Read the model definition and answer for the solid it produces. Units are mm, in the model's axes. A direction names the side the tool comes from. Round coordinates to 2 decimals unless told otherwise and drop trailing zeros. Write each loop counter-clockwise with the first axis right and the second up, starting at its lowest first coordinate (ties: lowest second). Pieces come first, ordered by that corner, then holes. Notation, with made-up numbers: (-1, 44) -> (41, 44) arc R9 ccw to (41, 60) -> close; hole circle Ø5 at (48.25, 29.5). An arc over 180 degrees is marked (long way). Return JSON: item names as keys, results as strings. Group by question number.
(1) The mould has two halves that part along Z. Classify faces 3 (the cylindrical face through (4.032, -6.324, -11.888)), 4 (the flat face through (2, 5, -0.1)), 5 (the cylindrical face through (6.87, -2.16, -3.49)), 6 (the cylindrical face through (6.87, -2.16, -20.49)): released by +Z, released by -Z, zero draft, split by the parting line, or undercut.
(2) For faces 1 (the flat face through (-2, 5, -23.9)), 2 (the cylindrical face through (-0.867, 3.905, -12.168)), determine the directions among +Z, -Z, +X, -X, +Y, -Y from which every point of the face is accessible in a straight line to the end or side of a thin tool.
(3) Straight lines are drawn through the part: line 1 (Y direction, x = 0, z = -23.95); line 2 (Y direction, x = -0.25, z = -6.5); line 3 (Z direction, x = -3, y = -4.5). For each, find the intervals that lie inside material, in ascending order.
(4) A cutting plane is placed at A-A on z = -18.25. Give the vertices of the cut face in (x, y), then the cut area to 3 significant figures.
(5) Given pin 1 (1 mm diameter, centred on x = 3.5, y = 5, fed in from -Z); pin 2 (1.5 mm diameter, centred on x = -2, z = -9, fed in from +Y); pin 3 (3 mm diameter, centred on x = -3.5, z = -11, fed in from +Y); pin 4 (6 mm diameter, centred on y = -5, z = -21.5, fed in from +X), each flat-ended and moving along its own axis, determine where each tip first touches the part or whether it passes through.
```python
from build123d import *

# Parameters (mm, degrees)
FILLET1_R = 0.2


with BuildPart() as part:
    # Sketch1 → Revolve1 (revolve)
    with BuildSketch(Plane(origin=(0, 0, 0), x_dir=(0, 0, -1), z_dir=(1, 0, 0)), mode=Mode.PRIVATE) as revolve1_sk:
        Polygon((0, 7.5), (0, 6.5), (0.1, 6.5), (0.1, 5), (0, 5), (0, 4), (24, 4), (24, 5), (23.9, 5), (23.9, 6.5), (24, 6.5), (24, 7.5), (21, 7.5), (21, 7.2), (20, 7.2), (20, 7.5), (4, 7.5), (4, 7.2), (3, 7.2), (3, 7.5), align=None)
    revolve(revolve1_sk.sketch.rotate(Axis((0, 0, 0), (0, 0, -1)), 90), axis=Axis((0, 0, 0), (0, 0, -1)))

    # Fillet1
    fillet1_edges = [part.edges().sort_by_distance(p)[0] for p in [
        (-7.5, 0, -24),
        (-7.5, 0, 0),
    ]]
    fillet(fillet1_edges, radius=FILLET1_R)


solid = part.part
```
Checks:
{
 "1": {"face 3": "zero draft", "face 4": "released by +Z", "face 5": "undercut", "face 6": "undercut"},
 "2": {"face 1": "-Z", "face 2": "+Z, -Z"},
 "3": {"line 1": "y = -7.43 to -6.5, -5 to -4, 4 to 5, 6.5 to 7.43", "line 2": "y = -7.5 to -3.99, 3.99 to 7.5", "line 3": "z = -23.9 to -0.1"},
 "4": {"outline": "circle Ø15 at (0, 0); hole circle Ø8 at (0, 0)", "area": "126 mm^2"},
 "5": {"pin 1": "stops at z = -24", "pin 2": "stops at y = 7.4", "pin 3": "stops at y = 7.23", "pin 4": "stops at x = 7.23"}
}
